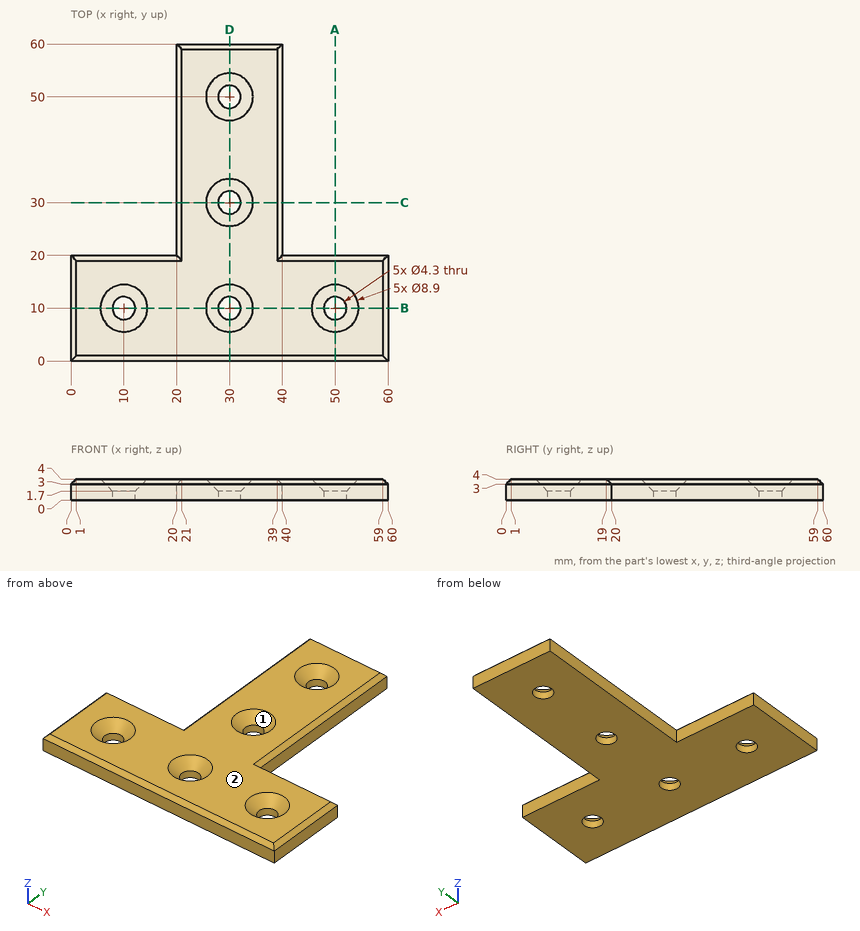
Here's the drawing with two shaded views (mm, measured from the low corner). I have some questions. Coordinates: 2 decimals unless noted, no trailing zeros. Write each loop counter-clockwise with the first axis right and the second up, starting at its lowest first coordinate (ties: lowest second). Pieces come first, ordered by that corner, then holes. Notation, with made-up numbers: M 61.25,-17.75 L 104.25,-17.75 A15 cw 104.25,1.25 Z; hole C -39,0.5 d7. An arc over 180 degrees is marked long. Write item = value, one per line. Start each with the question number.
Q1. Thinking about a two-plate mould opening in X: for the marked faces 1 and 2, which applies, released by +X, released by -X, zero draft, split by the parting line, or undercut?
Q2. I'm going to push flat-ended pins straight in: pin 1 (7 mm diameter, centred on x = 50, y = 10, fed in from +Z); pin 2 (1.5 mm diameter, centred on y = 50, z = 1.5, fed in from +X); pin 3 (0.9 mm diameter, centred on x = 14, z = 1, fed in from +Y). Where does each tip first touch, or does it pass through?
Q3. If we section it at A-A, the plane x = 50: Write out the boundary of the cut face in (y, z).
Q4. If we section it at C-C, the plane y = 30: Write out the boundary of the cut face in (x, z), then the cut area to 3 significant figures.
Q5. If we section it at B-B, the plane y = 10: Write out the boundary of the cut face in (x, z).
Q6. If I drill on L1, parallel to Y at x = 31, z = 2.85; L2, parallel to Y at x = 50, z = 1.2; L3, parallel to Y at x = 11.5, z = 3.1, over which ranges is the centre line in solid material (lowest first)? Write a range as [from, to].
Check sheet entries:
q1.face_1 = undercut
q1.face_2 = zero draft
q2.pin_1 = 3.05
q2.pin_2 = 40
q2.pin_3 = 20
q3.outline = M 0,0 L 7.85,0 L 7.85,1.7 L 5.55,4 L 1,4 L 0,3 Z; M 12.15,0 L 20,0 L 20,3 L 19,4 L 14.45,4 L 12.15,1.7 Z
q4.outline = M 20,0 L 27.85,0 L 27.85,1.7 L 25.55,4 L 21,4 L 20,3 Z; M 32.15,0 L 40,0 L 40,3 L 39,4 L 34.45,4 L 32.15,1.7 Z
q4.area = 56.5 mm²
q5.outline = M 0,0 L 7.85,0 L 7.85,1.7 L 5.55,4 L 1,4 L 0,3 Z; M 12.15,0 L 27.85,0 L 27.85,1.7 L 25.55,4 L 14.45,4 L 12.15,1.7 Z; M 32.15,0 L 47.85,0 L 47.85,1.7 L 45.55,4 L 34.45,4 L 32.15,1.7 Z; M 52.15,0 L 60,0 L 60,3 L 59,4 L 54.45,4 L 52.15,1.7 Z
q6.L1 = [0, 6.86], [13.14, 26.86], [33.14, 46.86], [53.14, 60]
q6.L2 = [0, 7.85], [12.15, 20]
q6.L3 = [0.1, 6.78], [13.22, 19.9]
